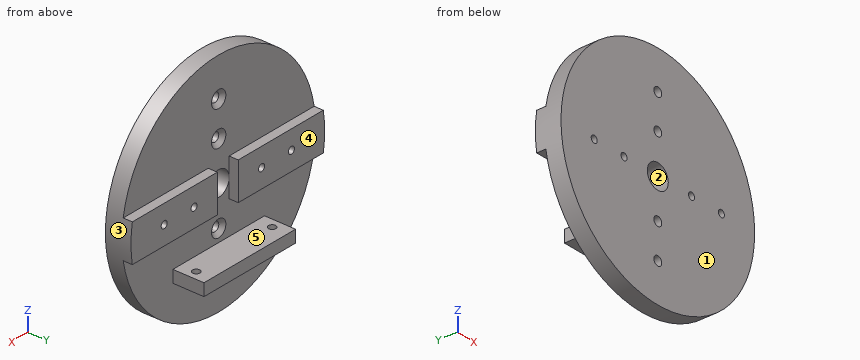
Autodesk Inventor part; units mm, degrees
ref_plane "YZ Plane" through (0, 0, 0) normal (1, 0, 0) x (0, 1, 0)
ref_plane "XZ Plane" through (0, 0, 0) normal (0, 1, 0) x (-1, 0, 0)
ref_plane "XY Plane" through (0, 0, 0) normal (0, 0, 1) x (1, 0, 0)
sketch "Sketch1" plane through (0, 0, 0) normal (0, 1, 0) x (-1, 0, 0)
  circle A0 centre (0, 0) radius 46.99
  line L0 (0, 0) -> (16.383, 0)
  line L1 (16.383, 0) -> (30.861, 0)
  line L2 (0, 0) -> (0, -16.383)
  line L3 (0, -16.383) -> (0, -30.861)
  line L4 (0, 0) -> (0, 16.383)
  line L5 (0, 16.383) -> (0, 30.861)
  line L6 (0, 0) -> (-16.383, 0)
  line L7 (-16.383, 0) -> (-30.861, 0)
  circle A1 centre (0, 30.861) radius 1.905
  circle A2 centre (30.861, 0) radius 1.4732
  circle A3 centre (0, -30.861) radius 1.905
  circle A4 centre (-30.861, 0) radius 1.4732
  circle A5 centre (-16.383, 0) radius 1.4732
  circle A6 centre (0, 16.383) radius 1.905
  circle A7 centre (16.383, 0) radius 1.4732
  circle A8 centre (0, -16.383) radius 1.905
  dimension "d0" = 93.98
  dimension "d1" = 16.383
  dimension "d2" = 14.478
  dimension "d3" = 16.383
  dimension "d4" = 14.478
  dimension "d5" = 16.383
  dimension "d6" = 14.478
  dimension "d7" = 16.383
  dimension "d8" = 14.478
  dimension "d9" = 3.81
  dimension "d10" = 2.9464
  dimension "d11" = 3.81
  dimension "d12" = 2.9464
  dimension "d13" = 2.9464
  dimension "d14" = 3.81
  dimension "d15" = 2.9464
  dimension "d16" = 3.81
extrude "Extrusion1" add sketch "Sketch1" along normal blind 6.858
sketch "Sketch2" plane through (0, 6.858, 0) normal (0, 1, 0) x (1, 0, 0)
  circle A0 centre (0, 0) radius 46.99
hole "Hole1" at (0, 6.858, 0) direction (0, -1, 0) diameter 10.16 depth 25.4 tip angle 118
sketch "Sketch3" plane through (0, 6.858, 0) normal (0, 1, 0) x (1, 0, 0)
  circle A0 centre (-16.383, 0) radius 1.4732
  circle A1 centre (16.383, 0) radius 1.4732
  circle A2 centre (30.861, 0) radius 1.4732
  circle A3 centre (-30.861, 0) radius 1.4732
  circle A4 centre (0, 0) radius 46.99
  line L0 (0, 0) -> (0, 7.8105)
  line L1 (0, 0) -> (0, -7.8105)
  line L2 (0, -7.8105) -> (46.3363, -7.8105)
  line L3 (0, 7.8105) -> (46.3363, 7.8105)
  line L4 (0, 7.8105) -> (-46.3363, 7.8105)
  line L5 (0, -7.8105) -> (-46.3363, -7.8105)
  line L6 (-5.08, -7.8105) -> (-5.08, 7.8105)
  line L7 (5.08, -7.8105) -> (5.08, 7.8105)
  dimension "d26" = 7.8105
  dimension "d27" = 7.8105
extrude "Extrusion2" add sketch "Sketch3" along normal blind 3.81 contours A4 L2 L7 L3 | L4 L6 L5 A4
chamfer "Chamfer1" distance 1.5875 angle 45 1 edges at (1.905, 6.858, 30.861)
chamfer "Chamfer2" distance 1.5875 angle 45 3 edges at (1.905, 6.858, 16.383) (1.905, 6.858, -16.383) (1.905, 6.858, -30.861)
sketch "Sketch4" plane through (0, 6.858, 0) normal (0, 1, 0) x (1, 0, 0)
  line L0 (0, 21.59) -> (22.225, 21.59)
  line L1 (0, 21.59) -> (-22.225, 21.59)
  line L2 (-22.225, 21.59) -> (-22.225, 26.67)
  line L3 (-22.225, 26.67) -> (22.225, 26.67)
  line L4 (22.225, 26.67) -> (22.225, 21.59)
  dimension "d37" = 22.225
  dimension "d38" = 22.225
  dimension "d39" = 5.08
extrude "Extrusion3" add sketch "Sketch4" along normal blind 12.954
sketch "Sketch5" plane through (22.225, 6.858, -26.67) normal (0, 0, -1) x (-1, 0, 0)
  line L0 (44.45, 0) -> (44.45, 12.954)
  line L1 (0, 0) -> (0, 12.954)
  line L2 (0, 6.477) -> (44.45, 6.477)
  line L3 (44.45, 6.477) -> (40.64, 6.477)
  line L4 (0, 6.477) -> (3.81, 6.477)
  circle A0 centre (3.81, 6.477) radius 1.524
  circle A1 centre (40.64, 6.477) radius 1.524
  point P0 (22.225, -6.858)
  dimension "d42" = 3.81
  dimension "d43" = 3.81
  dimension "d44" = 3.048
  dimension "d45" = 3.048
hole "Hole2" at (18.415, 13.335, -26.67) at (-18.415, 13.335, -26.67) direction (0, 0, 1) diameter 3.048 depth 25.4 tip angle 118
properties part number "Master Tablet and IR Mount"
Verification items for the finished model (mm, model axes). Face numbers are marked on the shaded views. A direction names the side the tool comes from. Coordinates: 2 decimals unless noted, no trailing zeros. Loops run counter-clockwise (first coordinate to the right, second up) from the corner with the lowest first, then second, coordinate; pieces in that order, holes last. Notation, with made-up numbers: (64, 57) -> (113, 57) arc R22 cw to (113, 86) -> close; hole circle Ø4 at (64, 12.25). An arc over 180 degrees is marked (long way). Write each question's results on one line, items separated by ' | '.
Item 1: Section check C-C, the plane x = -10. Enter the section's corners in (y, z).
Found:
outline: (0, -45.91) -> (6.86, -45.91) -> (6.86, -26.67) -> (19.81, -26.67) -> (19.81, -21.59) -> (6.86, -21.59) -> (6.86, -7.81) -> (10.67, -7.81) -> (10.67, 7.81) -> (6.86, 7.81) -> (6.86, 45.91) -> (0, 45.91) -> close
Item 2: Mould release check, pull along Z, two halves, no side actions. Record for the marked faces 1, 2 and 3: +Z half, -Z half, draft (parallel to the pull), parting line (faces both ways), or undercut.
Found:
face 1: draft | face 2: undercut | face 3: parting line
Item 3: Section check A-A, the plane x = 37. Enter the section's corners in (y, z).
Found:
outline: (0, -28.97) -> (6.86, -28.97) -> (6.86, -7.81) -> (10.67, -7.81) -> (10.67, 7.81) -> (6.86, 7.81) -> (6.86, 28.97) -> (0, 28.97) -> close
Item 4: Section check B-B, the plane x = 0. Count the separate pieces of the cut face and the enclosed holes in it, plus the area to 3 significant figures.
Found:
separate pieces: 6 | enclosed holes: 0 | area: 526 mm2
Item 5: Tool access check on the marked faces 4 and 5. Record the directions out of +Z, -Z, +X, -X, +Y, -Y that give a thin tool (end or side, any length) a straight path to the whole face; none if there is none.
Found:
face 4: +Z, +X, -X, +Y | face 5: +X, -X, +Y
Item 6: Material ranges on L1, parallel to Z at x = 0, y = 1.4; L2, parallel to Y at x = 27, z = -8.5; L3, parallel to Z at x = -36, y = 7.25, recorded low to high.
Found:
L1: z = -46.99 to -32.77, -28.96 to -18.29, -14.48 to -5.08, 5.08 to 14.48, 18.29 to 28.96, 32.77 to 46.99 | L2: y = 0 to 6.86 | L3: z = -7.81 to 7.81
Item 7: Gauge pin test, flat ends, axial feed: pin 1 (2.5 mm diameter, centred on x = -16.383, z = 0, fed in from -Y); pin 2 (3.5 mm diameter, centred on x = -30.861, z = 0, fed in from +Y); pin 3 (3 mm diameter, centred on y = 13.5, z = -28, fed in from +X) (3 decimals); pin 4 (10.5 mm diameter, centred on x = -9.5, y = 13, fed in from -Z). Record the tip position at first contact, or that the pin passes through.
Found:
pin 1: passes through | pin 2: stops at y = 10.67 | pin 3: stops at x = 22.225 | pin 4: stops at z = -26.67
